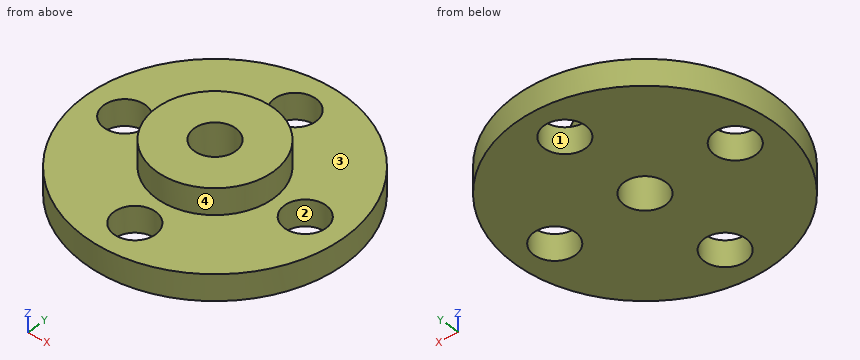
```python
from build123d import *

# Parameters (mm, degrees)
SKETCH_1_R          = 9.975
EXTRUDE_1_DEPTH     = 2
SKETCH_2_R          = 4.5
EXTRUDE_2_DEPTH     = 2
SKETCH_3_R          = 1.6
CUT_EXTRUDE_1_DEPTH = 15.662920923
SKETCH_4_R          = 1.6
CUT_EXTRUDE_2_DEPTH = 15.247850715


with BuildPart() as part:
    # ｽｹｯﾁ1 → ﾎﾞｽ - 押し出し1 (new body)
    with BuildSketch(Plane.XY):
        Circle(SKETCH_1_R)
    extrude(amount=EXTRUDE_1_DEPTH)

    # ｽｹｯﾁ2 → ﾎﾞｽ - 押し出し2 (add)
    with BuildSketch(Plane.XY.offset(2)):
        Circle(SKETCH_2_R)
    extrude(amount=EXTRUDE_2_DEPTH)

    # ｽｹｯﾁ3 → ｶｯﾄ - 押し出し1 (cut, through all)
    with BuildSketch(Plane.XY.offset(4)):
        Circle(SKETCH_3_R)
    extrude(amount=-CUT_EXTRUDE_1_DEPTH, mode=Mode.SUBTRACT)

    # ｽｹｯﾁ4 → ｶｯﾄ - 押し出し2 (cut, through all)
    with BuildSketch(Plane.XY.offset(2)):
        with Locations((0, 7)):
            Circle(SKETCH_4_R)
        with Locations((0, -7)):
            Circle(SKETCH_4_R)
        with Locations((-7, 0)):
            Circle(SKETCH_4_R)
        with Locations((7, 0)):
            Circle(SKETCH_4_R)
    extrude(amount=-CUT_EXTRUDE_2_DEPTH, mode=Mode.SUBTRACT)


solid = part.part
```
The listing builds one solid part. Answer for the finished solid, in the listing's coordinates (mm). Face numbers are marked on the shaded views. Give positions to 0.01 mm unless a question says otherwise; leave off trailing zeros. Order: outer loops, then holes, each group sorted by start corner. A loop starts at its lowest first (then second) coordinate and runs counter-clockwise, first axis right, second up. Notation, with made-up numbers: (-21.5, 58) -> (29.5, 58) arc R35 cw to (29.5, 92) -> close; hole circle Ø4 at (-38.75, 33). An arc over 180 degrees is marked (long way). Answer as a JSON object with one key per item and string values. Group by question number.
Item 1: The part is cut by section C-C on z = 1. Write down the section's boundary in (x, y) (3 decimals), and give its area (3 significant figures).
Item 2: The part is cut by section D-D on z = 2.9. Write down the section's boundary in (x, y), and give its area (3 significant figures).
Item 3: Determine the mould class of the marked faces 1, 2, 3 and 4 for opening direction X: pulls with the +X half, pulls with the -X half, needs draft (parallel to the pull), parting line crosses it, or undercut.
Item 4: The part is cut by section A-A on y = -7. Write down the section's boundary in (x, z).
Item 5: The part is cut by section B-B on x = 1. Write down the section's boundary in (y, z), and give its area (3 significant figures).
Item 6: Flat-ended cylindrical pins translate along their axes: pin 1 (3 mm diameter, centred on x = 0, y = -7, fed in from +Z); pin 2 (2 mm diameter, centred on x = 2, z = 1.5, fed in from +Y); pin 3 (1 mm diameter, centred on x = 5.5, y = 3, fed in from +Z); pin 4 (1.5 mm diameter, centred on y = 1, z = 1, fed in from -X). Find the tip coordinate at first contact, or state that the pin passes through.
Item 7: Consider L1, parallel to Y at x = 0, z = 0.5 (3 decimals); L2, parallel to X at y = 1.25, z = 1.7; L3, parallel to Z at x = -6.25, y = 3.5. Determine where each line is inside the solid, lowest interval first. Write a range as from..to.
Result set:
{
 "1": {"outline": "circle Ø19.95 at (0, 0); hole circle Ø3.2 at (-7, 0); hole circle Ø3.2 at (0, -7); hole circle Ø3.2 at (0, 0); hole circle Ø3.2 at (0, 7); hole circle Ø3.2 at (7, 0)", "area": "272 mm²"},
 "2": {"outline": "circle Ø9 at (0, 0); hole circle Ø3.2 at (0, 0)", "area": "55.6 mm²"},
 "3": {"face 1": "undercut", "face 2": "undercut", "face 3": "needs draft", "face 4": "parting line crosses it"},
 "4": {"outline": "(-7.11, 0) -> (-1.6, 0) -> (-1.6, 2) -> (-7.11, 2) -> close; (1.6, 0) -> (7.11, 0) -> (7.11, 2) -> (1.6, 2) -> close"},
 "5": {"outline": "(-9.92, 0) -> (-8.25, 0) -> (-8.25, 2) -> (-9.92, 2) -> close; (-5.75, 0) -> (-1.25, 0) -> (-1.25, 4) -> (-4.39, 4) -> (-4.39, 2) -> (-5.75, 2) -> close; (1.25, 0) -> (5.75, 0) -> (5.75, 2) -> (4.39, 2) -> (4.39, 4) -> (1.25, 4) -> close; (8.25, 0) -> (9.92, 0) -> (9.92, 2) -> (8.25, 2) -> close", "area": "37.3 mm²"},
 "6": {"pin 1": "through", "pin 2": "y = 9.92", "pin 3": "z = 2", "pin 4": "x = -9.97"},
 "7": {"L1": "-9.975..-8.6, -5.4..-1.6, 1.6..5.4, 8.6..9.975", "L2": "-9.9..-8, -6..-1, 1..6, 8..9.9", "L3": "0..2"}
}
